The figure shows three views and two pictorial views of one solid part (mm, origin at its lowest corner). Answer the questions. A direction names the side the tool comes from. Coordinates: 2 decimals unless noted, no trailing zeros. Order: outer loops, then holes, each group sorted by start corner. A loop starts at its lowest first (then second) coordinate and runs counter-clockwise, first axis right, second up. Notation, with made-up numbers: (37, 20.25) -> (62, 20.25) arc R16 ccw to (62, 36.25) -> close; hole circle Ø5 at (66.5, 14). An arc over 180 degrees is marked (long way). Use one line per item in the form item = value.
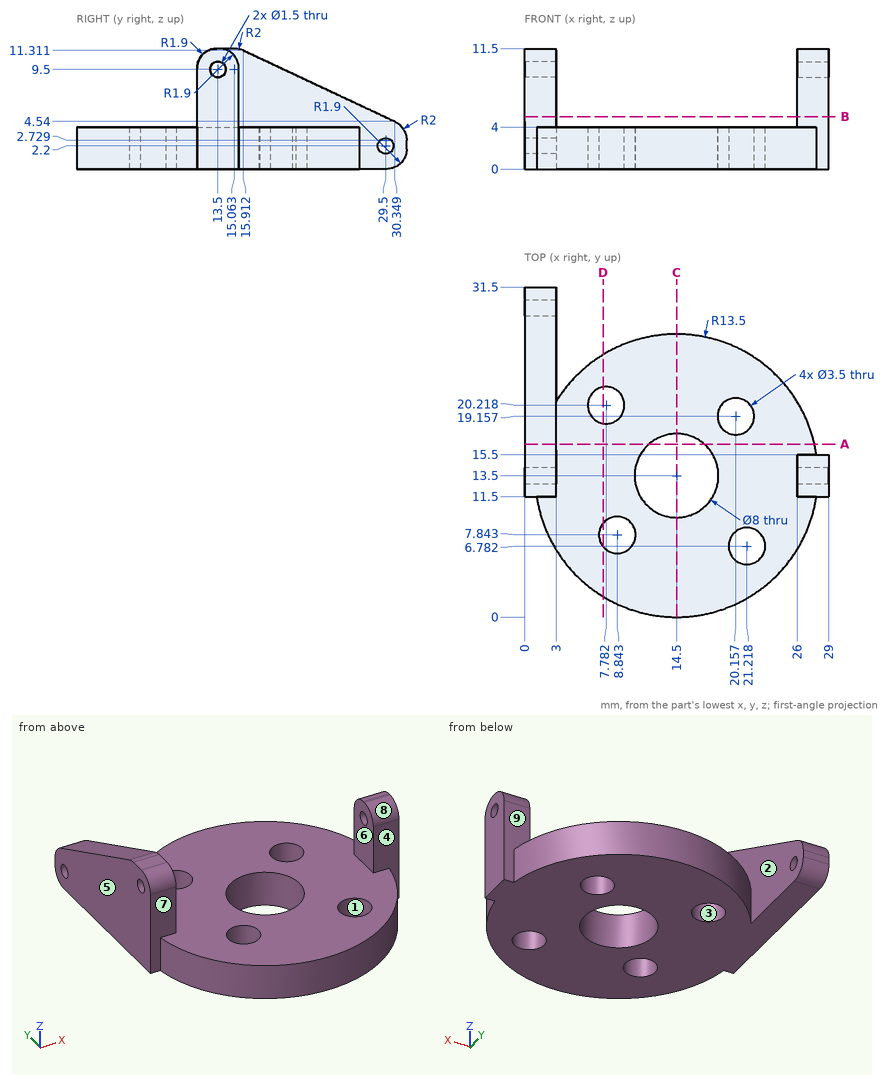
(1) Section A-A on y = 16.5 is taken. Write down the section's boundary in (x, z) (1 decimal), plus the area to 3 significant figures.
Data:
outline = (0, 0) -> (11.9, 0) -> (11.9, 4) -> (3, 4) -> (3, 11) -> (0, 11) -> close; (17.1, 0) -> (27.7, 0) -> (27.7, 4) -> (17.1, 4) -> close
area = 111 mm²
(2) Section D-D on x = 7.5 is taken. Write down the section's boundary in (y, z) (1 decimal).
Data:
outline = (2, 0) -> (6.7, 0) -> (6.7, 4) -> (2, 4) -> close; (9, 0) -> (18.5, 0) -> (18.5, 4) -> (9, 4) -> close; (21.9, 0) -> (25, 0) -> (25, 4) -> (21.9, 4) -> close
(3) Straight lines are drawn through the part: line 1 along Y through (x, z) = (20.5, 3.75) (1 decimal); line 2 along X through (y, z) = (19, 3.25) (1 decimal); line 3 along Y through (x, z) = (13.25, 3.75). For each, find the intervals that lie inside material, in ascending order.
Data:
line_1 = 1.4 to 5.2, 8.4 to 17.4, 20.9 to 25.6
line_2 = 0 to 6.5, 9 to 18.4, 21.9 to 26.8
line_3 = 0.06 to 9.7, 17.3 to 26.94
(4) Section C-C on x = 14.5 is taken. Write down the section's boundary in (y, z).
Data:
outline = (0, 0) -> (9.5, 0) -> (9.5, 4) -> (0, 4) -> close; (17.5, 0) -> (27, 0) -> (27, 4) -> (17.5, 4) -> close
(5) Section B-B on z = 5 is taken. Write down the section's boundary in (x, y).
Data:
outline = (0, 11.5) -> (3, 11.5) -> (3, 29.37) -> (0, 29.37) -> close; (26, 11.5) -> (29, 11.5) -> (29, 15.5) -> (26, 15.5) -> close
(6) Which of the six approach directions +Z, -Z, +X, -X, +Y, -Y give full straight-line access (tool end or side, diameter ignored) to the marked faces 5, 6, 7, 8 and 9?
Data:
face_5 = +Z, -Z, -X, +Y, -Y
face_6 = +Z, +Y, -Y
face_7 = +Z, -X, -Y
face_8 = +Z, +X, -X, -Y
face_9 = +Z, +X, +Y
(7) Each of these flat-tipped pins is pushed along its axis until it touches: P1, Ø4, axis at x = 22.5, z = 8, coming from the -Y side; P2, Ø9, axis at x = 14.5, y = 13.5, coming from the +Z side; P3, Ø2.5, axis at x = 27, z = 6, coming from the +Y side; P4, Ø4, axis at x = 8.84, y = 7.84, coming from the -Z side. Where does it stop, or does it pass through?
Data:
P1 = through
P2 = 4
P3 = 15.5
P4 = 0
(8) The mould has two halves that part along Y. Classify the marked faces 1, 2, 3 and 4: released by +Y, released by -Y, zero draft, split by the parting line, or undercut.
Data:
face_1 = undercut
face_2 = zero draft
face_3 = undercut
face_4 = released by -Y
